Verification items for the finished model (mm, model axes). A direction names the side the tool comes from. Coordinates: 2 decimals unless noted, no trailing zeros. Order: outer loops, then holes, each group sorted by start corner. A loop starts at its lowest first (then second) coordinate and runs counter-clockwise, first axis right, second up. Notation, with made-up numbers: M 20.25,4 L 67.25,4 A24 ccw 67.25,32 Z; hole C -18,13.5 d1. An arc over 180 degrees is marked long. Return JSON: item names as keys, results as strings. Group by question number.
Q1. Section check B-B, the plane y = 16. Enter the section's corners in (x, z) (3 decimals).
Q2. Access from +Z, -Z, +X, -X, +Y, -Y to the whole of each face (thin tool, end or side, straight path). Record for faces 1 (the face through (2.072, 23.835, 1.174)), 2 (the face through (0.69, 9.4, 3.1)), 3 (the face through (0, 0, 0)).
Q3. Go/stop test with flat-tipped pins: pin 1 Ø4 at (x, y) = (3.5, 7) entering from -Z; pin 2 Ø1.5 at (x, z) = (-3, 2) entering from -Y; pin 3 Ø1.4 at (x, z) = (0, -1) entering from +Y (3 decimals). Record where each tip stops, or that it passes through.
Q4. Thickness scan on probe 1 along Y at (x, z) = (1.5, 0.75) (3 decimals); probe 2 along Y at (x, z) = (-3.5, 0.75); probe 3 along Z at (x, y) = (1, 24.25). Record the ranges inside material, lowest first.
Q5. Mould release check, pull along X, two halves, no side actions. Record for faces 4 (the face through (-2.05, 23.83, 1.21)), 5 (the face through (1, 19.05, -4)), 6 (the face through (-3.78, 21.98, -2.9)), 7 (the face through (2.05, 23.83, -1.21)): pulls with the +X half, pulls with the -X half, needs draft (parallel to the pull), parting line crosses it, or undercut.
Autodesk Inventor part; units mm, degrees
ref_plane "YZ Plane" through (0, 0, 0) normal (1, 0, 0) x (0, 1, 0)
ref_plane "XZ Plane" through (0, 0, 0) normal (0, 1, 0) x (-1, 0, 0)
ref_plane "XY Plane" through (0, 0, 0) normal (0, 0, 1) x (1, 0, 0)
sketch "Sketch1" plane through (0, 0, 0) normal (0, 1, 0) x (-1, 0, 0)
  circle A0 centre (0, 0) radius 3.175
  dimension "d0" = 6.35
extrude "Extrusion1" add sketch "Sketch1" along normal blind 19.05
sketch "Sketch2" plane through (0, 19.05, 0) normal (0, 1, 0) x (1, 0, 0)
  circle A0 centre (0, 0) radius 3.175
  circle A1 centre (0, 0) radius 4.7625
  dimension "d3" = 9.525
extrude "Extrusion2" add sketch "Sketch2" along normal blind 6.35 contours A0 | A1
sketch "Sketch3" plane through (0, 25.4, 0) normal (0, 1, 0) x (1, 0, 0)
  circle A0 centre (0, 0) radius 4.7625
  line L0 (-1.3748, 2.3812) -> (1.3748, 2.3813)
  line L1 (1.3748, 2.3813) -> (2.7496, 0)
  line L2 (2.7496, 0) -> (1.3748, -2.3813)
  line L3 (1.3748, -2.3813) -> (-1.3748, -2.3813)
  line L4 (-1.3748, -2.3813) -> (-2.7496, 0)
  line L5 (-2.7496, 0) -> (-1.3748, 2.3812)
  dimension "d6" = 4.7625
extrude "Extrusion3" cut sketch "Sketch3" against normal blind 3.175 contours L0 L1 L2 L3 L4 L5
fillet "Fillet1" radius 0.3969 3 edges at (3.175, 19.05, 0) (-4.7625, 25.4, 0) (3.175, 0, 0)
properties part number "Bolt_0.25_20_0.75len_SocketHead" material "Stainless Steel, Austenitic"
Numbers:
{
 "1": {"outline": "C 0,0 d6.35"},
 "2": {"face 1": "+Y", "face 2": "-Y", "face 3": "+Z, -Z, +X, -X, -Y"},
 "3": {"pin 1": "stops at z = -2.8", "pin 2": "stops at y = 0.01", "pin 3": "stops at y = 22.225"},
 "4": {"probe 1": "y = 0 to 22.225", "probe 2": "y = 19.05 to 25.4", "probe 3": "z = -4.66 to -2.38, 2.38 to 4.66"},
 "5": {"face 4": "undercut", "face 5": "needs draft", "face 6": "parting line crosses it", "face 7": "undercut"}
}
